Source: CAD feature listing. Evaluate the final solid. Frame: model axes, mm. A direction names the side the tool comes from. Coordinates: 2 decimals unless noted, no trailing zeros. Order: outer loops, then holes, each group sorted by start corner. A loop starts at its lowest first (then second) coordinate and runs counter-clockwise, first axis right, second up.
```python
from build123d import *

# Parameters (mm, degrees)
SKETCH1_W                 = 43.18
SKETCH1_H                 = 25.4
BASE_DEPTH                = 37.592
SIDECHAMFER_SIZE          = 12.7
BACKCHAMFERS_SIZE         = 6.35
SKETCH2_W                 = 12.065
SKETCH2_H                 = 11.938
LINACTSLOT_DEPTH          = 51.24387091
MOUTINGHOLES_D            = 2.7051
MOUTINGHOLES_DEPTH        = 14.478
MOUTINGHOLES_TIP          = 0.81269403
MOTORSLOT_DEPTH           = 51.24387091
MOTORMOUNTINGHOLES2_D     = 2.2606
MOTORMOUNTINGHOLES2_DEPTH = 11.43
MOTORMOUNTINGHOLES2_TIP   = 0.679152758


with BuildPart() as part:
    # Sketch1 → Base (new body)
    with BuildSketch(Plane(origin=(0, 0, 0), x_dir=(1, 0, 0), z_dir=(0, 1, 0))):
        Rectangle(SKETCH1_W, SKETCH1_H)
    extrude(amount=BASE_DEPTH)

    # SideChamfer
    sidechamfer_edges = [part.edges().sort_by_distance(p)[0] for p in [
        (21.59, 0, 0),
    ]]
    chamfer(sidechamfer_edges, length=SIDECHAMFER_SIZE)

    # BackChamfers
    backchamfers_edges = [part.edges().sort_by_distance(p)[0] for p in [
        (21.59, 25.146, 12.7),
        (-21.59, 18.796, 12.7),
    ]]
    chamfer(backchamfers_edges, length=BACKCHAMFERS_SIZE)

    # Sketch2 → LinActSlot (cut, through all)
    with BuildSketch(Plane.XY.offset(12.7)):
        with Locations((0, 31.623)):
            Rectangle(SKETCH2_W, SKETCH2_H)
    extrude(amount=-LINACTSLOT_DEPTH, mode=Mode.SUBTRACT)

    # MoutingHoles
    with Locations(Plane(origin=(14.160350453, 37.592, 8.373414988), x_dir=(-1, 0, 0), z_dir=(0, 1, 0))):
        with Locations((1.460350453, -4.563414988), (26.860350453, -4.563414988)):
            Hole(MOUTINGHOLES_D / 2, depth=MOUTINGHOLES_DEPTH)
            with Locations((0, 0, -(MOUTINGHOLES_DEPTH + MOUTINGHOLES_TIP / 2))):  # 118° drill point
                Cone(0, MOUTINGHOLES_D / 2, MOUTINGHOLES_TIP, mode=Mode.SUBTRACT)

    # Sketch11 → MotorSlot (cut, through all)
    with BuildSketch(Plane(origin=(0, 0, -12.7), x_dir=(-1, 0, 0), z_dir=(0, 0, -1))):
        with BuildLine():
            Line((15.875, 5.08), (15.875, 5.715))
            ThreePointArc((15.875, 5.715), (13.085192091, 12.450192091), (6.35, 15.24))
            Line((6.35, 15.24), (5.08, 15.24))
            ThreePointArc((5.08, 15.24), (-1.655192091, 12.450192091), (-4.445, 5.715))
            Line((-4.445, 5.715), (-4.445, 5.08))
            Line((-4.445, 5.08), (-4.445, 0))
            Line((-4.445, 0), (15.875, 0))
            Line((15.875, 0), (15.875, 5.08))
        make_face()
    extrude(amount=-MOTORSLOT_DEPTH, mode=Mode.SUBTRACT)

    # MotorMountingHoles2
    with Locations(Plane(origin=(0, 0, -12.7), x_dir=(-1, 0, 0), z_dir=(0, 0, -1))):
        with Locations((18.215, 5.715), (-6.785, 5.715)):
            Hole(MOTORMOUNTINGHOLES2_D / 2, depth=MOTORMOUNTINGHOLES2_DEPTH)
            with Locations((0, 0, -(MOTORMOUNTINGHOLES2_DEPTH + MOTORMOUNTINGHOLES2_TIP / 2))):  # 118° drill point
                Cone(0, MOTORMOUNTINGHOLES2_D / 2, MOTORMOUNTINGHOLES2_TIP, mode=Mode.SUBTRACT)


solid = part.part
```
1. Section query A-A on y = 8.5. Return loops of the section in (x, z), plus the area to 3 significant figures.
Findings:
outline: (-21.59, -12.7) - (-15.46, -12.7) - (-15.46, 12.48) - (-21.59, 6.35) - close; (4.03, -12.7) - (17.39, -12.7) - (17.39, 10.55) - (15.24, 12.7) - (4.03, 12.7) - close
area: 473 mm2
2. Ray query, line 1 (X direction, y = 27.5, z = 3.81); line 2 (X direction, y = 27, z = 1); line 3 (Y direction, x = -17.5, z = -5.5). Return the intervals inside material, ascending.
Findings:
line 1: x = -21.59 to -14.05, -11.35 to -6.03, 6.03 to 11.35, 14.05 to 21.59
line 2: x = -21.59 to -6.03, 6.03 to 21.59
line 3: y = 0 to 4.84, 6.59 to 37.59
3. Access query for faces 1 (the face through (4.445, 3, 0)), 2 (the face through (11.35, 30.25, 3.87)), 3 (the face through (0, 25.654, 0)), 4 (the face through (-18.46, 18.53, 9.48)), 5 (the face through (5.952, 6.479, -6.905)). Directions: +Z, -Z, +X, -X, +Y, -Y. A direction counts if a zero-diameter tool reaches every point of the face in a straight line with its end or side. Return the directions, or none.
Findings:
face 1: +Z, -Z, -Y
face 2: +Y
face 3: +Z, -Z, +Y
face 4: +Z, -X, +Y, -Y
face 5: -Z
4. Section query C-C on z = -7.75. Count the separate pieces of the cut face and the enclosed holes in it, plus the area to 3 significant figures.
Findings:
separate pieces: 1
enclosed holes: 2
area: 1,120 mm2
5. Pin query (flat end, axial travel): P1, Ø2, axis at x = -18.215, y = 5.715, coming from the +Z side (3 decimals); P2, Ø2, axis at x = 12.7, z = 3.81, coming from the -Y side; P3, Ø1.8, axis at x = 6.785, y = 5.715, coming from the -Z side. Return the tip coordinate at first contact, or that it passes through.
Findings:
P1: stops at z = 10.725
P2: stops at y = 2.81
P3: stops at z = -1.13
6. Section query B-B on y = 24. Return loops of the section in (x, z), plus the area to 3 significant figures.
Findings:
outline: (-21.59, -12.7) - (21.59, -12.7) - (21.59, 6.35) - (15.24, 12.7) - (-15.24, 12.7) - (-21.59, 6.35) - close; hole circle Ø2.71 at (-12.7, 3.81); hole circle Ø2.71 at (12.7, 3.81)
area: 1,040 mm2
7. Draft query along Y for faces 6 (the face through (7, 0, 0)), 7 (the face through (-18.07, 5.85, -0.71)), 8 (the face through (0, 19, -12.7)). Return one class per face: released by +Y, released by -Y, zero draft, split by the parting line, or undercut.
Findings:
face 6: released by -Y
face 7: undercut
face 8: zero draft
